```python
from build123d import *

# Parameters (mm, degrees)
SKETCH1_W            = 124.4
SKETCH1_H            = 111.7
BOSS_EXTRUDE1_DEPTH  = 15.65
FILLET1_R            = 2
SKETCH4_W            = 115
SKETCH4_H            = 102.3
CUT_EXTRUDE1_DEPTH   = 2
SKETCH5_W            = 112
SKETCH5_H            = 99.3
CUT_EXTRUDE2_DEPTH   = 3
SKETCH10_W           = 7
SKETCH10_H           = 7
BOSS_EXTRUDE2_DEPTH  = 3
BOSS_EXTRUDE5_DEPTH  = 35
FILLET3_R            = 6
SKETCH32_W           = 114.7
SKETCH32_H           = 2.7
SKETCH32_W_2         = 2.7
SKETCH32_H_2         = 102.3
CUT_EXTRUDE7_DEPTH   = 3.5
SKETCH29_W           = 27
SKETCH29_H           = 3.5
CUT_EXTRUDE8_DEPTH   = 112.7
SKETCH34_W           = 1
SKETCH34_H           = 31.5
CUT_EXTRUDE9_DEPTH   = 2
SKETCH39_W           = 124.4
SKETCH39_H           = 111.7
CUT_EXTRUDE14_DEPTH  = 8.65
SKETCH40_W           = 10.736913624
SKETCH40_H           = 4.7
BOSS_EXTRUDE8_DEPTH  = 7
SKETCH42_W           = 6.036913624
SKETCH42_H           = 2.116828075
BOSS_EXTRUDE9_DEPTH  = 7
SKETCH43_W           = 2
SKETCH43_H           = 3.979386742
BOSS_EXTRUDE10_DEPTH = 7
SKETCH44_W           = 10.013933806
SKETCH44_H           = 10.028001726
BOSS_EXTRUDE11_DEPTH = 7
SKETCH45_R           = 1.1
CUT_EXTRUDE15_DEPTH  = 8
SKETCH46_W           = 2
SKETCH46_H           = 2
BOSS_EXTRUDE12_DEPTH = 7
SKETCH47_W           = 2
SKETCH47_H           = 2
BOSS_EXTRUDE13_DEPTH = 7
SKETCH48_W           = 10
SKETCH48_H           = 10
BOSS_EXTRUDE14_DEPTH = 7
SKETCH49_R           = 1.1
SKETCH49_W           = 6.036913624
SKETCH49_H           = 6.816828075
CUT_EXTRUDE18_DEPTH  = 7
SKETCH50_W           = 8
SKETCH50_H           = 10
BOSS_EXTRUDE17_DEPTH = 7
SKETCH51_W           = 5.24842793
SKETCH51_H           = 4.514776714
BOSS_EXTRUDE18_DEPTH = 7
SKETCH52_W           = 2
SKETCH52_H           = 10
CUT_EXTRUDE19_DEPTH  = 7
SKETCH53_W           = 10.013933806
SKETCH53_H           = 10.028001726
CUT_EXTRUDE20_DEPTH  = 7
SKETCH54_W           = 8
SKETCH54_H           = 10
BOSS_EXTRUDE19_DEPTH = 7
SKETCH55_W           = 8
SKETCH55_H           = 10
BOSS_EXTRUDE20_DEPTH = 7
SKETCH56_R           = 1.1
CUT_EXTRUDE21_DEPTH  = 7
SKETCH57_R           = 1.1
CUT_EXTRUDE22_DEPTH  = 7
SKETCH58_R           = 1.1
CUT_EXTRUDE23_DEPTH  = 7
SKETCH59_R           = 1.1
CUT_EXTRUDE24_DEPTH  = 7
SKETCH61_W           = 20.033048375
SKETCH61_H           = 15
SKETCH61_W_2         = 20.00121795
BOSS_EXTRUDE22_DEPTH = 8
SKETCH64_R           = 1.1
CUT_EXTRUDE27_DEPTH  = 51
SKETCH65_R           = 3
CUT_EXTRUDE28_DEPTH  = 2


with BuildPart() as part:
    # Sketch1 → Boss-Extrude1 (new body)
    with BuildSketch(Plane(origin=(0, 0, 0), x_dir=(1, 0, 0), z_dir=(0, 1, 0))):
        with Locations((62.2, 55.85)):
            Rectangle(SKETCH1_W, SKETCH1_H)
    extrude(amount=BOSS_EXTRUDE1_DEPTH)

    # Fillet1
    fillet1_edges = [part.edges().sort_by_distance(p)[0] for p in [
        (0, 7.825, -111.7),
        (124.4, 7.825, -111.7),
        (124.4, 7.825, 0),
        (0, 7.825, 0),
    ]]
    fillet(fillet1_edges, radius=FILLET1_R)

    # Sketch4 → Cut-Extrude1 (cut)
    with BuildSketch(Plane(origin=(0, 15.65, 0), x_dir=(1, 0, 0), z_dir=(0, 1, 0))):
        with Locations((62.2, 55.85)):
            Rectangle(SKETCH4_W, SKETCH4_H)
    extrude(amount=-CUT_EXTRUDE1_DEPTH, mode=Mode.SUBTRACT)

    # Sketch5 → Cut-Extrude2 (cut)
    with BuildSketch(Plane(origin=(0, 13.65, 0), x_dir=(1, 0, 0), z_dir=(0, 1, 0))):
        with Locations((62.2, 55.85)):
            Rectangle(SKETCH5_W, SKETCH5_H)
    extrude(amount=-CUT_EXTRUDE2_DEPTH, mode=Mode.SUBTRACT)

    # Sketch10 → Boss-Extrude2 (add)
    with BuildSketch(Plane(origin=(0, 10.65, 0), x_dir=(1, 0, 0), z_dir=(0, 1, 0))):
        with Locations((9.7, 102)):
            Rectangle(SKETCH10_W, SKETCH10_H)
        with Locations((9.7, 9.7)):
            Rectangle(SKETCH10_W, SKETCH10_H)
        with Locations((114.7, 102)):
            Rectangle(SKETCH10_W, SKETCH10_H)
        with Locations((114.7, 9.7)):
            Rectangle(SKETCH10_W, SKETCH10_H)
    extrude(amount=BOSS_EXTRUDE2_DEPTH)

    # Sketch27 → Boss-Extrude5 (add)
    with BuildSketch(Plane(origin=(0, 15.65, 0), x_dir=(1, 0, 0), z_dir=(0, 1, 0))):
        Polygon((5, 110.35), (119.4, 110.35), (119.4, 108.316244658), (5, 108.35), align=None)
    extrude(amount=BOSS_EXTRUDE5_DEPTH)

    # Fillet3
    fillet3_edges = [part.edges().sort_by_distance(p)[0] for p in [
        (111.2, 12.15, -13.2),
        (13.2, 12.15, -98.5),
        (13.2, 12.15, -13.2),
        (111.2, 12.15, -98.5),
    ]]
    fillet(fillet3_edges, radius=FILLET3_R)

    # Sketch32 → Cut-Extrude7 (cut)
    with BuildSketch(Plane(origin=(0, 15.65, 0), x_dir=(1, 0, 0), z_dir=(0, 1, 0))):
        with Locations((62.2, 2.35)):
            Rectangle(SKETCH32_W, SKETCH32_H)
        with Locations((2.35, 55.85)):
            Rectangle(SKETCH32_W_2, SKETCH32_H_2)
        with Locations((122.05, 55.85)):
            Rectangle(SKETCH32_W_2, SKETCH32_H_2)
    extrude(amount=-CUT_EXTRUDE7_DEPTH, mode=Mode.SUBTRACT)

    # Sketch29 → Cut-Extrude8 (cut, through all)
    with BuildSketch(Plane(origin=(0, 0, -111.7), x_dir=(-1, 0, 0), z_dir=(0, 0, -1))):
        with Locations((-34.4, 17.4)):
            Rectangle(SKETCH29_W, SKETCH29_H)
    extrude(amount=-CUT_EXTRUDE8_DEPTH, mode=Mode.SUBTRACT)

    # Sketch34 → Cut-Extrude9 (cut)
    with BuildSketch(Plane(origin=(0, 15.65, 0), x_dir=(1, 0, 0), z_dir=(0, 1, 0))):
        with Locations((4.2, 82.55)):
            Rectangle(SKETCH34_W, SKETCH34_H)
    extrude(amount=-CUT_EXTRUDE9_DEPTH, mode=Mode.SUBTRACT)

    # Sketch39 → Cut-Extrude14 (cut)
    with BuildSketch(Plane(origin=(0, 0, 0), x_dir=(-1, 0, 0), z_dir=(0, -1, 0))):
        with Locations((-62.2, 55.85)):
            Rectangle(SKETCH39_W, SKETCH39_H)
    extrude(amount=-CUT_EXTRUDE14_DEPTH, mode=Mode.SUBTRACT)

    # Sketch40 → Boss-Extrude8 (add)
    with BuildSketch(Plane(origin=(0, 15.65, 0), x_dir=(1, 0, 0), z_dir=(0, 1, 0))):
        with Locations((-0.668456812, 2.35)):
            Rectangle(SKETCH40_W, SKETCH40_H)
    extrude(amount=-BOSS_EXTRUDE8_DEPTH)

    # Sketch42 → Boss-Extrude9 (add)
    with BuildSketch(Plane(origin=(0, 15.65, 0), x_dir=(1, 0, 0), z_dir=(0, 1, 0))):
        with Locations((-3.018456812, 5.758414037)):
            Rectangle(SKETCH42_W, SKETCH42_H)
    extrude(amount=-BOSS_EXTRUDE9_DEPTH)

    # Sketch43 → Boss-Extrude10 (add)
    with BuildSketch(Plane(origin=(0, 15.65, 0), x_dir=(1, 0, 0), z_dir=(0, 1, 0))):
        with Locations((123.4, 1.989693371)):
            Rectangle(SKETCH43_W, SKETCH43_H)
    extrude(amount=-BOSS_EXTRUDE10_DEPTH)

    # Sketch44 → Boss-Extrude11 (add)
    with BuildSketch(Plane(origin=(0, 15.65, 0), x_dir=(1, 0, 0), z_dir=(0, 1, 0))):
        with Locations((129.406966903, 5.014000863)):
            Rectangle(SKETCH44_W, SKETCH44_H)
    extrude(amount=-BOSS_EXTRUDE11_DEPTH)

    # Sketch45 → Cut-Extrude15 (cut, through all)
    with BuildSketch(Plane(origin=(0, 15.65, 0), x_dir=(1, 0, 0), z_dir=(0, 1, 0))):
        with Locations((129.4, 5)):
            Circle(SKETCH45_R)
    extrude(amount=-CUT_EXTRUDE15_DEPTH, mode=Mode.SUBTRACT)

    # Sketch46 → Boss-Extrude12 (add)
    with BuildSketch(Plane(origin=(0, 15.65, 0), x_dir=(1, 0, 0), z_dir=(0, 1, 0))):
        with Locations((123.4, 110.7)):
            Rectangle(SKETCH46_W, SKETCH46_H)
    extrude(amount=-BOSS_EXTRUDE12_DEPTH)

    # Sketch47 → Boss-Extrude13 (add)
    with BuildSketch(Plane(origin=(0, 15.65, 0), x_dir=(1, 0, 0), z_dir=(0, 1, 0))):
        with Locations((1, 110.7)):
            Rectangle(SKETCH47_W, SKETCH47_H)
    extrude(amount=-BOSS_EXTRUDE13_DEPTH)

    # Sketch48 → Boss-Extrude14 (add)
    with BuildSketch(Plane(origin=(0, 15.65, 0), x_dir=(1, 0, 0), z_dir=(0, 1, 0))):
        with Locations((-5, 106.7)):
            Rectangle(SKETCH48_W, SKETCH48_H)
    extrude(amount=-BOSS_EXTRUDE14_DEPTH)

    # Sketch49 → Cut-Extrude18 (cut)
    with BuildSketch(Plane(origin=(0, 15.65, 0), x_dir=(1, 0, 0), z_dir=(0, 1, 0))):
        with Locations((-5, 106.7)):
            Circle(SKETCH49_R)
        with Locations((-3.018456812, 3.408414038)):
            Rectangle(SKETCH49_W, SKETCH49_H)
    extrude(amount=-CUT_EXTRUDE18_DEPTH, mode=Mode.SUBTRACT)

    # Sketch50 → Boss-Extrude17 (add)
    with BuildSketch(Plane(origin=(0, 15.65, 0), x_dir=(1, 0, 0), z_dir=(0, 1, 0))):
        with Locations((-4, 5)):
            Rectangle(SKETCH50_W, SKETCH50_H)
    extrude(amount=-BOSS_EXTRUDE17_DEPTH)

    # Sketch51 → Boss-Extrude18 (add)
    with BuildSketch(Plane(origin=(0, 15.65, 0), x_dir=(1, 0, 0), z_dir=(0, 1, 0))):
        with Locations((-4.818404413, 107.053945145)):
            Rectangle(SKETCH51_W, SKETCH51_H)
    extrude(amount=-BOSS_EXTRUDE18_DEPTH)

    # Sketch52 → Cut-Extrude19 (cut)
    with BuildSketch(Plane(origin=(0, 15.65, 0), x_dir=(1, 0, 0), z_dir=(0, 1, 0))):
        with Locations((-9, 106.7)):
            Rectangle(SKETCH52_W, SKETCH52_H)
    extrude(amount=-CUT_EXTRUDE19_DEPTH, mode=Mode.SUBTRACT)

    # Sketch53 → Cut-Extrude20 (cut)
    with BuildSketch(Plane(origin=(0, 15.65, 0), x_dir=(1, 0, 0), z_dir=(0, 1, 0))):
        with Locations((129.406966903, 5.014000863)):
            Rectangle(SKETCH53_W, SKETCH53_H)
    extrude(amount=-CUT_EXTRUDE20_DEPTH, mode=Mode.SUBTRACT)

    # Sketch54 → Boss-Extrude19 (add)
    with BuildSketch(Plane(origin=(0, 15.65, 0), x_dir=(1, 0, 0), z_dir=(0, 1, 0))):
        with Locations((128.4, 5)):
            Rectangle(SKETCH54_W, SKETCH54_H)
    extrude(amount=-BOSS_EXTRUDE19_DEPTH)

    # Sketch55 → Boss-Extrude20 (add)
    with BuildSketch(Plane(origin=(0, 15.65, 0), x_dir=(1, 0, 0), z_dir=(0, 1, 0))):
        with Locations((128.4, 106.7)):
            Rectangle(SKETCH55_W, SKETCH55_H)
    extrude(amount=-BOSS_EXTRUDE20_DEPTH)

    # Sketch56 → Cut-Extrude21 (cut)
    with BuildSketch(Plane(origin=(0, 15.65, 0), x_dir=(1, 0, 0), z_dir=(0, 1, 0))):
        with Locations((-3.1, 106.7)):
            Circle(SKETCH56_R)
    extrude(amount=-CUT_EXTRUDE21_DEPTH, mode=Mode.SUBTRACT)

    # Sketch57 → Cut-Extrude22 (cut)
    with BuildSketch(Plane(origin=(0, 15.65, 0), x_dir=(1, 0, 0), z_dir=(0, 1, 0))):
        with Locations((-3.1, 5)):
            Circle(SKETCH57_R)
    extrude(amount=-CUT_EXTRUDE22_DEPTH, mode=Mode.SUBTRACT)

    # Sketch58 → Cut-Extrude23 (cut)
    with BuildSketch(Plane(origin=(0, 15.65, 0), x_dir=(1, 0, 0), z_dir=(0, 1, 0))):
        with Locations((127.5, 5)):
            Circle(SKETCH58_R)
    extrude(amount=-CUT_EXTRUDE23_DEPTH, mode=Mode.SUBTRACT)

    # Sketch59 → Cut-Extrude24 (cut)
    with BuildSketch(Plane(origin=(0, 15.65, 0), x_dir=(1, 0, 0), z_dir=(0, 1, 0))):
        with Locations((127.5, 106.7)):
            Circle(SKETCH59_R)
    extrude(amount=-CUT_EXTRUDE24_DEPTH, mode=Mode.SUBTRACT)

    # Sketch61 → Boss-Extrude22 (add)
    with BuildSketch(Plane.XZ.offset(-8.65)):
        with Locations((62.216524188, -84.35)):
            Rectangle(SKETCH61_W, SKETCH61_H)
        with Locations((62.200608975, -27.35)):
            Rectangle(SKETCH61_W_2, SKETCH61_H)
    extrude(amount=BOSS_EXTRUDE22_DEPTH)

    # Sketch64 → Cut-Extrude27 (cut, through all)
    with BuildSketch(Plane(origin=(0, 0.65, 0), x_dir=(-1, 0, 0), z_dir=(0, -1, 0))):
        with Locations((-62.216524187, 84.35)):
            Circle(SKETCH64_R)
        with Locations((-62.200608975, 27.35)):
            Circle(SKETCH64_R)
    extrude(amount=-CUT_EXTRUDE27_DEPTH, mode=Mode.SUBTRACT)

    # Sketch65 → Cut-Extrude28 (cut)
    with BuildSketch(Plane(origin=(0, 10.65, 0), x_dir=(1, 0, 0), z_dir=(0, 1, 0))):
        with Locations((62.200608975, 27.35)):
            Circle(SKETCH65_R)
        with Locations((62.216524187, 84.35)):
            Circle(SKETCH65_R)
    extrude(amount=-CUT_EXTRUDE28_DEPTH, mode=Mode.SUBTRACT)


solid = part.part
```
Could you check a few things on this model? Use its own coordinates, in mm. A direction names the side the tool comes from. Coordinates: 2 decimals unless noted, no trailing zeros. Write each loop counter-clockwise with the first axis right and the second up, starting at its lowest first coordinate (ties: lowest second). Pieces come first, ordered by that corner, then holes. Notation, with made-up numbers: (21.25, 10) -> (64.25, 10) arc R24 cw to (64.25, 23) -> close; hole circle Ø6 at (81.25, 54). An arc over 180 degrees is marked (long way). Write item = value, one per line. Start each with the question number.
(1) Will these pins go through, and if not, where does the flat tip stop? pin 1 (6 mm diameter, centred on x = 26.5, z = -24.5, fed in from +Y); pin 2 (10 mm diameter, centred on x = 94.5, y = 34, fed in from -Z); pin 3 (2 mm diameter, centred on x = 62.22, z = -84.35, fed in from -Y); pin 4 (3 mm diameter, centred on x = 88, z = -2, fed in from +Y).
(2) I need wall thicknesses on line 1 (Z direction, x = 127.5, y = 13.5); line 2 (X direction, y = 13.25, z = -106.7); line 3 (Z direction, x = 59, y = 15). Which ranges of each line are inside material? Lowest first, please. Write a range as [from, to].
(3) We'd pull the mould along Z, two halves only. Please class faces 1 (the face through (62, 5, -76.85)), 2 (the face through (64, 8.65, -84)), 3 (the face through (62, 5, -19.85)), 4 (the face through (132.4, 12, -5)): released by +Z, released by -Z, zero draft, split by the parting line, or undercut.
(4) I want a section at C-C (x = 113.5). Please give me the cut outline in (y, z), plus the area to 3 significant figures.
(5) I want a section at A-A (z = -57). Please give me the cut outline in (x, y).
(6) I want a section at B-B (y = 35). Please give me the cut outline in (x, z).
(7) Which directions (+Z, -Z, +X, -X, +Y, -Y) give clear straight access to the entire face, cutting with the end or side of a thin tool? Please do faces 5 (the face through (6.2, 12, -55)), 6 (the face through (-8, 12, -107)), 7 (the face through (52.2, 5, -27)), 8 (the face through (128, 12, -101.7)), 9 (the face through (61, 12, 0)).
Result set:
q1.pin_1 = 10.65
q1.pin_2 = -110.35
q1.pin_3 = through
q1.pin_4 = 15.65
q2.line_1 = [-111.7, -107.8], [-105.6, -101.7], [-10, -6.1], [-3.9, 0]
q2.line_2 = [-8, -4.2], [-2, 1], [3.7, 120.7], [123.4, 126.4], [128.6, 132.4]
q2.line_3 = [-111.7, -107], [-4.7, -3.7], [-1, 0]
q3.face_1 = undercut
q3.face_2 = undercut
q3.face_3 = released by +Z
q3.face_4 = zero draft
q4.outline = (8.65, -111.7) -> (15.65, -111.7) -> (15.65, -110.35) -> (50.65, -110.35) -> (50.65, -108.32) -> (15.65, -108.32) -> (15.65, -107) -> (13.65, -107) -> (13.65, -99.78) -> (10.65, -99.78) -> (10.65, -11.92) -> (13.65, -11.92) -> (13.65, -4.7) -> (15.65, -4.7) -> (15.65, -3.7) -> (12.15, -3.7) -> (12.15, -1) -> (15.65, -1) -> (15.65, 0) -> (8.65, 0) -> close
q4.area = 375 mm2
q5.outline = (0, 8.65) -> (124.4, 8.65) -> (124.4, 15.65) -> (123.4, 15.65) -> (123.4, 12.15) -> (120.7, 12.15) -> (120.7, 15.65) -> (119.7, 15.65) -> (119.7, 13.65) -> (118.2, 13.65) -> (118.2, 10.65) -> (6.2, 10.65) -> (6.2, 13.65) -> (4.7, 13.65) -> (4.7, 15.65) -> (3.7, 15.65) -> (3.7, 12.15) -> (1, 12.15) -> (1, 15.65) -> (0, 15.65) -> close
q6.outline = (5, -110.35) -> (119.4, -110.35) -> (119.4, -108.32) -> (5, -108.35) -> close
q7.face_5 = +Y
q7.face_6 = +Z, -Z, -X, +Y, -Y
q7.face_7 = +Z, -Z, -X, -Y
q7.face_8 = +X, +Y, -Y
q7.face_9 = +Z, +X, -X, +Y, -Y
